The listing builds one solid part. Answer for the finished solid, in the listing's coordinates (mm). Face numbers are marked on the shaded views. A direction names the side the tool comes from. Give positions to 0.01 mm unless a question says otherwise; leave off trailing zeros. Order: outer loops, then holes, each group sorted by start corner. A loop starts at its lowest first (then second) coordinate and runs counter-clockwise, first axis right, second up. Notation, with made-up numbers: (18, 26) - (49, 26) arc R22 ccw to (49, 63) - close; hole circle Ø3 at (3.5, 74). An arc over 180 degrees is marked (long way). Answer as a JSON object with one key per item and string values. Group by question number.
Q1. A cutting plane is placed at A-A, the plane x = 0. Count the separate pieces of the cut face and the enclosed holes in it, and give its area (3 significant figures).
Q2. The mould has two halves that part along X. Classify the marked faces 1, 2 and 3: released by +X, released by -X, zero draft, split by the parting line, or undercut.
Q3. For the marked faces 4, 5 and 6, determine the directions among +Z, -Z, +X, -X, +Y, -Y from which every point of the face is accessible in a straight line to the end or side of a thin tool.
Q4. Consider line 1 (Y direction, x = 0, z = 20.25); line 2 (X direction, y = -11.5, z = 15); line 3 (Y direction, x = -16, z = 16.75). Determine where each line is inside the solid, lowest interval first.
Q5. A cutting plane is placed at C-C, the plane y = -27.5. Give the vertices of the cut face in (x, z).
Q6. Given pin 1 (1.3 mm diameter, centred on x = 1, z = 16.5, fed in from -Y); pin 2 (2 mm diameter, centred on x = 13, z = 8.5, fed in from +Y); pin 3 (5 mm diameter, centred on y = -25.5, z = 19, fed in from +X); pin 4 (4 mm diameter, centred on x = 0, y = 0, fed in from +Z), each flat-ended and moving along its own axis, determine where each tip first touches the part or whether it passes through.
Q7. A cutting plane is placed at B-B, the plane z = 21.75. Give the vertices of the cut face in (x, y), and give its area (3 significant figures).
from build123d import *

# Parameters (mm, degrees)
SKETCH1_R           = 31.75
BOSS_EXTRUDE1_DEPTH = 25.4
SKETCH3_R           = 21.59
CUT_EXTRUDE1_DEPTH  = 7.62
SKETCH4_R           = 21.59
CUT_EXTRUDE2_DEPTH  = 12.7
CUT_EXTRUDE3_DEPTH  = 13.7
BOSS_EXTRUDE2_DEPTH = 5.08
CIRPATTERN1_COUNT   = 6
CUT_EXTRUDE5_DEPTH  = 2.54
SKETCH8_R           = 2.159
CUT_EXTRUDE6_DEPTH  = 2.54
CUT_EXTRUDE7_DEPTH  = 1.6764


with BuildPart() as part:
    # Sketch1 → Boss-Extrude1 (new body)
    with BuildSketch(Plane.XY):
        Circle(SKETCH1_R)
    extrude(amount=BOSS_EXTRUDE1_DEPTH)

    # Sketch3 → Cut-Extrude1 (cut)
    with BuildSketch(Plane.XY.offset(25.4)):
        Circle(SKETCH3_R)
    extrude(amount=-CUT_EXTRUDE1_DEPTH, mode=Mode.SUBTRACT)

    # Sketch4 → Cut-Extrude2 (cut)
    with BuildSketch(Plane(origin=(0, 0, 0), x_dir=(-1, 0, 0), z_dir=(0, 0, -1))):
        Circle(SKETCH4_R)
    extrude(amount=-CUT_EXTRUDE2_DEPTH, mode=Mode.SUBTRACT)

    # Sketch5 → Cut-Extrude3 (cut, through all)
    with BuildSketch(Plane(origin=(0, 0, 12.7), x_dir=(-1, 0, 0), z_dir=(0, 0, -1))):
        with BuildLine():
            Line((-3.169774213, 7.622175309), (-4.990334321, 20.025058542))
            ThreePointArc((-4.990334321, 20.025058542), (-12.706659311, -16.261833088), (20.6375, 0))
            ThreePointArc((20.6375, 0), (16.238120297, 12.736948436), (4.915648471, 20.043522803))
            Line((4.915648471, 20.043522803), (3.767056418, 7.345359824))
            ThreePointArc((3.767056418, 7.345359824), (7.044220174, 4.303950178), (8.255, 0))
            ThreePointArc((8.255, 0), (-4.581404745, -6.867004847), (-3.169774213, 7.622175309))
        make_face()
        with BuildLine():
            ThreePointArc((-3.245486062, 20.380707212), (-4.121747911, 20.221711115), (-4.990334321, 20.025058542))
            Line((-4.990334321, 20.025058542), (-3.169774213, 7.622175309))
            ThreePointArc((-3.169774213, 7.622175309), (-2.322085611, 7.921675543), (-1.446854472, 8.127215829))
            Line((-1.446854472, 8.127215829), (-3.245486062, 20.380707212))
        make_face()
        with BuildLine():
            ThreePointArc((3.194434326, 20.388771311), (-0.025842356, 20.63748382), (-3.245486062, 20.380707212))
            Line((-3.245486062, 20.380707212), (-1.446854472, 8.127215829))
            ThreePointArc((-1.446854472, 8.127215829), (0.320434302, 8.248778507), (2.072967036, 7.990483882))
            Line((2.072967036, 7.990483882), (3.194434326, 20.388771311))
        make_face()
        with BuildLine():
            ThreePointArc((4.915648471, 20.043522803), (4.058714067, 20.234456908), (3.194434326, 20.388771311))
            Line((3.194434326, 20.388771311), (2.072967036, 7.990483882))
            ThreePointArc((2.072967036, 7.990483882), (2.937773774, 7.714564813), (3.767056418, 7.345359824))
            Line((3.767056418, 7.345359824), (4.915648471, 20.043522803))
        make_face()
    extrude(amount=-CUT_EXTRUDE3_DEPTH, mode=Mode.SUBTRACT)

    # Sketch5<3> → Boss-Extrude2 (add)
    with BuildSketch(Plane(origin=(0, 0, 12.7), x_dir=(-1, 0, 0), z_dir=(0, 0, -1))):
        with BuildLine():
            ThreePointArc((-3.245486062, 20.380707212), (-4.121747911, 20.221711115), (-4.990334321, 20.025058542))
            Line((-4.990334321, 20.025058542), (-3.169774213, 7.622175309))
            ThreePointArc((-3.169774213, 7.622175309), (-2.322085611, 7.921675543), (-1.446854472, 8.127215829))
            Line((-1.446854472, 8.127215829), (-3.245486062, 20.380707212))
        make_face()
        with BuildLine():
            ThreePointArc((4.915648471, 20.043522803), (4.058714067, 20.234456908), (3.194434326, 20.388771311))
            Line((3.194434326, 20.388771311), (2.072967036, 7.990483882))
            ThreePointArc((2.072967036, 7.990483882), (2.937773774, 7.714564813), (3.767056418, 7.345359824))
            Line((3.767056418, 7.345359824), (4.915648471, 20.043522803))
        make_face()
    boss_extrude2 = extrude(amount=-BOSS_EXTRUDE2_DEPTH)

    # CirPattern1: Boss-Extrude2 ×6 about axis
    cirpattern1_axis = Axis((0, 0, 0), (0, 0, 1))
    for i in range(1, CIRPATTERN1_COUNT):
        add(boss_extrude2.rotate(cirpattern1_axis, i * 360 / CIRPATTERN1_COUNT))

    # Sketch7 → Cut-Extrude5 (cut)
    with BuildSketch(Plane.XY.offset(17.78)):
        Polygon((6.35, 0), (3.175, 5.499261314), (-3.175, 5.499261314), (-6.35, 0), (-3.175, -5.499261314), (3.175, -5.499261314), align=None)
    extrude(amount=-CUT_EXTRUDE5_DEPTH, mode=Mode.SUBTRACT)

    # Sketch8 → Cut-Extrude6 (cut)
    with BuildSketch(Plane.XY.offset(15.24)):
        Circle(SKETCH8_R)
    extrude(amount=-CUT_EXTRUDE6_DEPTH, mode=Mode.SUBTRACT)

    # Sketch9 → Cut-Extrude7 (cut)
    with BuildSketch(Plane(origin=(0, 0, 12.7), x_dir=(-1, 0, 0), z_dir=(0, 0, -1))):
        Polygon((7.020387337, 0), (2.169418994, 6.676785124), (-5.679612663, 4.126480142), (-5.679612663, -4.126480142), (2.169418994, -6.676785124), align=None)
    extrude(amount=-CUT_EXTRUDE7_DEPTH, mode=Mode.SUBTRACT)


solid = part.part
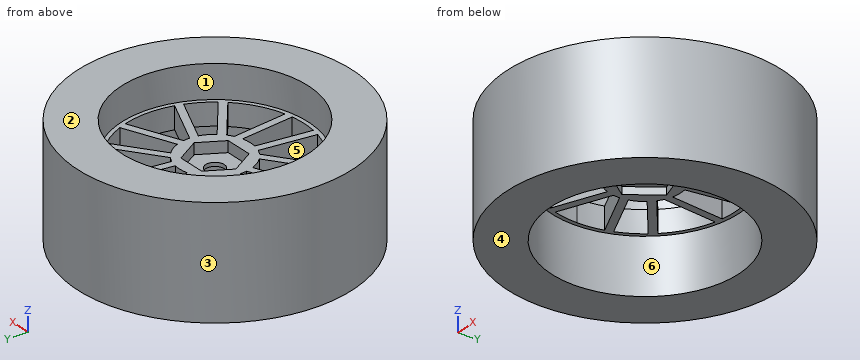
Reply:
{
 "1": {"separate pieces": "4", "enclosed holes": "0", "area": "558 mm^2"},
 "2": {"face 1": "undercut", "face 2": "zero draft", "face 3": "split by the parting line"},
 "3": {"face 4": "-Z, +X, -X, +Y, -Y", "face 5": "+Z, -Z", "face 6": "-Z"},
 "4": {"line 1": "y = -31.75 to -21.59, 21.59 to 31.75", "line 2": "x = -29.59 to -17.14, -13.99 to -10.96, -3.74 to -1.94, 2.39 to 4.14, 11.26 to 14.13, 17.14 to 29.59", "line 3": "y = -27.42 to -12.92, -6.08 to -4.17, 4 to 5.92, 12.98 to 27.42"},
 "5": {"outline": "(-15.87, 0) - (15.87, 0) - (15.87, 25.4) - (-15.87, 25.4) - close"},
 "6": {"pin 1": "stops at y = -31.75", "pin 2": "stops at y = 29.39", "pin 3": "stops at x = 21.89", "pin 4": "passes through"},
 "7": {"outline": "circle Ø63.5 at (0, 0); hole circle Ø43.18 at (0, 0)", "area": "1,700 mm^2"}
}
